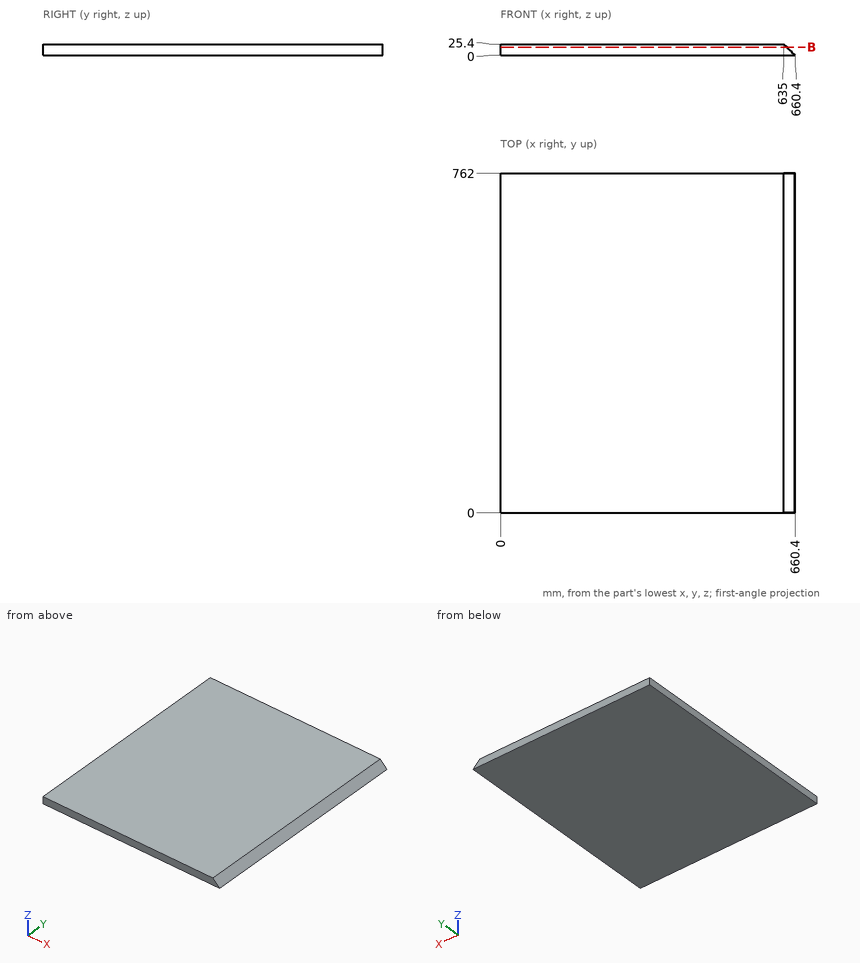
Geometry check sheet. Reference: drawing and pictorial views, mm from the part's lowest x, y, z. Round coordinates to 2 decimals unless told otherwise and drop trailing zeros. Order: outer loops, then holes, each group sorted by start corner. A loop starts at its lowest first (then second) coordinate and runs counter-clockwise, first axis right, second up. Notation, with made-up numbers: M -23.75,13 L -5.75,13 A29 ccw -5.75,44 Z; hole C -18,89 d5. An arc over 180 degrees is marked long. One line per item, written item: value. Start each with the question number.
1. Scan lines: line 1 along X through (y, z) = (700, 14.5); line 2 along X through (y, z) = (176, 22). Record each from-to range of solid material in increasing order.
2. Section check B-B on z = 18.5. Enter the section's corners in (x, y).
3. Gauge pin test, flat ends, axial feed: P1, Ø5, axis at y = 311.5, z = 15.5, coming from the +X side; P2, Ø1.5, axis at y = 584, z = 5.5, coming from the +X side. Record the tip position at first contact, or that the pin passes through.
Results found:
1. line 1: 0 to 645.9
1. line 2: 0 to 638.4
2. outline: M 0,0 L 641.9,0 L 641.9,762 L 0,762 Z
3. P1: x = 647.4
3. P2: x = 655.65
